Can you work these out from the model? Positions are in its coordinate system, mm. A direction names the side the tool comes from. Coordinates: 2 decimals unless noted, no trailing zeros. Write each loop counter-clockwise with the first axis right and the second up, starting at its lowest first coordinate (ties: lowest second). Pieces come first, ordered by that corner, then holes. Notation, with made-up numbers: (76, -39.75) -> (90, -39.75) arc R12 ccw to (90, -18.75) -> close; hole circle Ø9 at (80.5, -9). An arc over 180 degrees is marked (long way). Use one line per item in the form item = value.
```python
from build123d import *

# Parameters (mm, degrees)
EXTRUDE_1_DEPTH     = 14
SKETCH_2_R          = 25
EXTRUDE_2_DEPTH     = 30
SKETCH_3_R          = 12.5
CUT_EXTRUDE_1_DEPTH = 78.786850529
SKETCH_4_W          = 15.8
SKETCH_4_H          = 8
CUT_EXTRUDE_2_DEPTH = 78.786850529
SWEEP_2_PROFILE_R   = 2.5


with BuildPart() as part:
    # 草图1 → 凸台-拉伸1 (new body)
    with BuildSketch(Plane.XY):
        with BuildLine():
            add(Edge.make_bspline(
                [(33, 0), (32.994684587, 0.450024215), (32.984052078, 1.350215217), (32.901076258, 2.698653645), (32.772860205, 4.043927251), (32.597324571, 5.384974816), (32.378634546, 6.721198171), (32.032078752, 8.498284254), (31.501703341, 10.710471336), (30.726699331, 13.347427223), (29.820422985, 15.978337375), (28.78376894, 18.611676644), (27.610273888, 21.254339279), (26.515182854, 23.45103287), (25.5574803, 25.211343802), (24.789016632, 26.54270045), (23.972675772, 27.874149931), (23.105472148, 29.203671357), (22.184421782, 30.528688408), (21.206602984, 31.846069432), (20.16924743, 33.152137052), (19.069811985, 34.442677822), (17.90606236, 35.712977232), (16.676140858, 36.957852112), (15.37863945, 38.17170453), (14.012657383, 39.348574759), (12.57785829, 40.48221221), (11.07450942, 41.566141858), (9.503524234, 42.593753741), (7.866477955, 43.558375054), (6.165627296, 44.453366408), (4.403908588, 45.272204934), (2.584926869, 46.008571066), (0.712936618, 46.656438122), (-1.207193797, 47.210150802), (-3.170021946, 47.66451179), (-5.169590122, 48.014834863), (-7.19948183, 48.257032362), (-9.252895705, 48.387650153), (-11.322721226, 48.403921527), (-13.401619953, 48.303802916), (-15.482112157, 48.085992666), (-17.556663385, 47.74994839), (-19.617771107, 47.295872816), (-21.658056561, 46.724726957), (-23.670342116, 46.038176688), (-25.647738102, 45.238585056), (-27.583709079, 44.328944976), (-29.472149374, 43.312844419), (-31.307433374, 42.194386964), (-33.084472119, 40.978136682), (-34.798745182, 39.669031546), (-36.446339426, 38.272314352), (-38.023943914, 36.793434836), (-39.528922958, 35.238009279), (-40.959078807, 33.611599403), (-42.313460643, 31.920114124), (-43.589311507, 30.167983471), (-44.793272704, 28.364572965), (-45.530637058, 27.121554401), (-45.899346, 26.5)],
                knots=[0, 0, 0, 0, 0.011720528, 0.02344477, 0.035174471, 0.046912746, 0.058664172, 0.070434849, 0.094064277, 0.117883715, 0.141995125, 0.166516265, 0.191571891, 0.217283663, 0.230421312, 0.243762401, 0.257317187, 0.271094269, 0.285100438, 0.299340704, 0.313818209, 0.328534322, 0.343488665, 0.358679258, 0.374102619, 0.38975391, 0.405627105, 0.421715168, 0.438010208, 0.454503662, 0.471186473, 0.488049229, 0.505082314, 0.522276079, 0.539620899, 0.557107331, 0.574726161, 0.592468467, 0.610325686, 0.6282896, 0.646352393, 0.664506599, 0.682745118, 0.701061152, 0.719448204, 0.737900044, 0.756410636, 0.774974145, 0.7935849, 0.812237383, 0.830926227, 0.84964623, 0.86839239, 0.887159977, 0.90594454, 0.924742047, 0.943548942, 0.962362269, 0.981179768, 1, 1, 1, 1], degree=3))
            add(Edge.make_bspline(
                [(-45.899346, 26.5), (-46.183686014, 25.99658476), (-46.752365912, 24.989754507), (-47.542151603, 23.44514535), (-48.284558357, 21.877468697), (-48.974312895, 20.285818041), (-49.611879734, 18.672591924), (-50.196252541, 17.039331265), (-50.726892215, 15.387834686), (-51.203206677, 13.719857757), (-51.62469458, 12.037190136), (-51.990895237, 10.341632673), (-52.301444487, 8.635001114), (-52.555908827, 6.919122788), (-52.754388224, 5.195835615), (-52.895284113, 3.466984365), (-52.98361346, 1.734420848), (-52.994537821, 0.578140181), (-53, 0)],
                knots=[0, 0, 0, 0, 0.062500008, 0.124999987, 0.187499996, 0.249999999, 0.312499987, 0.374999994, 0.437500002, 0.500000019, 0.562500001, 0.625000006, 0.687500007, 0.75000001, 0.812500019, 0.874999996, 0.937500015, 1, 1, 1, 1], degree=3))
            add(Edge.make_bspline(
                [(-53, 0), (-52.994536306, -0.578068365), (-52.983610487, -1.734039205), (-52.890921769, -3.465687653), (-52.737459804, -5.192153917), (-52.514830205, -6.910368406), (-52.221750153, -8.616869483), (-51.855756316, -10.30788244), (-51.415431279, -11.979386603), (-50.899814435, -13.627185589), (-50.308555585, -15.246972675), (-49.641851525, -16.834390924), (-48.90046009, -18.385099751), (-48.085659908, -19.894826006), (-47.199233749, -21.359419817), (-46.243441559, -22.77490659), (-45.220979977, -24.137526422), (-44.134954865, -25.443781463), (-42.988839739, -26.690470176), (-41.786431369, -27.874717783), (-40.531812023, -28.994003994), (-39.22930277, -30.046187837), (-37.883420895, -31.029524247), (-36.498828408, -31.94267376), (-35.08029367, -32.784716601), (-33.632637068, -33.55514713), (-32.160696249, -34.253885921), (-30.669272011, -34.881258756), (-29.163092884, -35.437998224), (-27.646770009, -35.925222878), (-26.124761473, -36.344421792), (-24.601335518, -36.69743659), (-23.080535449, -36.986424819), (-21.566151621, -37.21384479), (-20.06169318, -37.382416012), (-18.570364754, -37.495089115), (-17.09504745, -37.555010185), (-15.63828303, -37.565478254), (-14.202260945, -37.529911258), (-12.788815604, -37.451808758), (-11.399408098, -37.334697574), (-9.594924838, -37.132882108), (-7.403548822, -36.80259903), (-4.857653491, -36.301470095), (-2.413691345, -35.722805964), (-0.064581352, -35.086952206), (2.19985327, -34.409599534), (4.391499881, -33.700962662), (6.522577444, -32.965335838), (8.60383086, -32.200414937), (10.643647529, -31.398673827), (12.643577343, -30.542836156), (14.606977568, -29.624742426), (15.869373093, -28.927262542), (16.5, -28.578838)],
                knots=[0, 0, 0, 0, 0.018617485, 0.037229627, 0.055835032, 0.074431523, 0.093016392, 0.111586604, 0.130138962, 0.148670157, 0.167176824, 0.185655535, 0.204102805, 0.22251502, 0.240888411, 0.259219008, 0.277502562, 0.295734481, 0.313909833, 0.332023234, 0.350068877, 0.368040428, 0.385931136, 0.403733696, 0.421440373, 0.439042968, 0.456532892, 0.473901167, 0.491138559, 0.508235601, 0.525182699, 0.541970207, 0.558588573, 0.575028394, 0.591280583, 0.607336484, 0.623187988, 0.638827665, 0.654248924, 0.669446162, 0.68441483, 0.699151658, 0.727921526, 0.755761391, 0.782700659, 0.808796619, 0.834133633, 0.858819493, 0.882978406, 0.906741052, 0.93023242, 0.953559502, 0.976800752, 1, 1, 1, 1], degree=3))
            add(Edge.make_bspline(
                [(16.5, -28.578838), (17.116689929, -28.207079649), (18.350069625, -27.463563045), (20.10262845, -26.197892511), (21.774178875, -24.828826667), (23.35112871, -23.351084244), (24.828450291, -21.773980361), (26.19935355, -20.10346697), (27.458095264, -18.346914058), (28.599248007, -16.511783882), (29.617940435, -14.605950878), (30.509791163, -12.637572777), (31.27104422, -10.615077714), (31.898195971, -8.547128331), (32.389483458, -6.442578551), (32.739354772, -4.310440562), (32.959177295, -2.15984452), (32.986392432, -0.719948155), (33, 0)],
                knots=[0, 0, 0, 0, 0.062500006, 0.124999996, 0.187499992, 0.249999998, 0.312500003, 0.374999999, 0.437499989, 0.499999995, 0.562499988, 0.625000012, 0.687500008, 0.750000012, 0.812499988, 0.875000009, 0.937500007, 1, 1, 1, 1], degree=3))
        make_face()
    extrude(amount=EXTRUDE_1_DEPTH)

    # 草图2 → 凸台-拉伸2 (add)
    with BuildSketch(Plane.XY):
        with Locations(Location((0, 0, 0), (0, 0, 180))):
            Circle(SKETCH_2_R)
    extrude(amount=EXTRUDE_2_DEPTH)

    # 草图3 → 切除-拉伸1 (cut, through all)
    with BuildSketch(Plane.XY):
        Circle(SKETCH_3_R)
    extrude(amount=CUT_EXTRUDE_1_DEPTH, mode=Mode.SUBTRACT)

    # 草图4 → 切除-拉伸2 (cut, through all)
    with BuildSketch(Plane.XY):
        with Locations((7.9, 0)):
            Rectangle(SKETCH_4_W, SKETCH_4_H)
    extrude(amount=CUT_EXTRUDE_2_DEPTH, mode=Mode.SUBTRACT)

    # 切除-扫描2: sweep along a curve in space
    with BuildLine() as sweep_2_path:
        Line((-1, 0, 22), (26, 0, 22))
    # 切除-扫描2 profile (on start of the path) → 切除-扫描2 (sweep, cut)
    with BuildSketch(Plane(origin=(-1, 0, 22), x_dir=(0, 0, 1), z_dir=(1, 0, 0))):
        Circle(SWEEP_2_PROFILE_R)
    sweep(path=sweep_2_path.line, mode=Mode.SUBTRACT)


solid = part.part
```
Q1. Thinking about a two-plate mould opening in Z: for faces 1 (the flat face through (14, -4, 15)), 2 (the flat face through (-19, 5, 0)), 3 (the flat face through (5.9, -11.5, 30)), 4 (the cylindrical face through (20.5, -0.1, 19.5)), which applies, released by +Z, released by -Z, zero draft, split by the parting line, or undercut?
Return value:
face_1 = zero draft
face_2 = released by -Z
face_3 = released by +Z
face_4 = undercut
Q2. Suppose I cut it at A-A (z = 26). Write out the boundary of the cut face in (x, y), then the cut area to 3 significant figures.
Return value:
outline = circle Ø50 at (0, 0); hole (11.84, -4) -> (15.8, -4) -> (15.8, 4) -> (11.84, 4) arc R12.5 ccw (long way) to start
area = 1,440 mm2
Q3. If I drill on line 1 (X direction, y = 0, z = 11.5); line 2 (Z direction, x = 21, y = 0); line 3 (X direction, y = 0.5, z = 18) (3 decimals), over which ranges is the centre line in solid material (lowest first)? Write a range as from..to.
Return value:
line_1 = -53..-12.5, 15.8..33
line_2 = 0..19.5, 24.5..30
line_3 = -24.995..-12.49, 15.8..24.995
Q4. For faces 5 (the cylindrical face through (-23.846, -7.509, 21.888)), 6 (the flat face through (14, 4, 15)), which set-ups out of +Z, -Z, +X, -X, +Y, -Y let a thin tool reach every point of the face, with its end or its side?
Return value:
face_5 = +Z
face_6 = +Z, -Z
Q5. Will these pins go through, and if not, where does the flat tip stop? pin 1 (12 mm diameter, centred on y = -12, z = 8.5, fed in from -X); pin 2 (4.5 mm diameter, centred on x = 14.5, z = 20, fed in from +Y); pin 3 (3 mm diameter, centred on y = -9.5, z = 4.5, fed in from -X); pin 4 (8 mm diameter, centred on x = -26, y = 2, fed in from -Z).
Return value:
pin_1 = -52.63
pin_2 = 21.79
pin_3 = -52.32
pin_4 = 0
